Can you work these out from the model? Positions are in its coordinate system, mm. A direction names the side the tool comes from. Give positions to 0.01 mm unless a question says otherwise; leave off trailing zeros. Write each loop counter-clockwise with the first axis right and the second up, starting at its lowest first coordinate (ties: lowest second). Pieces come first, ordered by that corner, then holes.
1. Thinking about a two-plate mould opening in Y: for faces 1 (the cylindrical face through (2.22, 219.61, 609.44)), 2 (the flat face through (-1, 29.618, 320)), 3 (the flat face through (80, 96, 320)), 4 (the flat face through (-1, 274.618, 609)), which applies, pulls with the +Y half, pulls with the -Y half, needs draft (parallel to the pull), parting line crosses it, or undercut?
2. Suppose I cut it at B-B (y = 201.5). Please give me the cut outline in (x, z), and give its area (3 significant figures).
3. Suppose I cut it at A-A (x = 22.5). Please give me the cut outline in (y, z).
4. I'm going to push flat-ended pins straight in: pin 1 (6.5 mm diameter, centred on y = 89.62, z = 140, fed in from +X); pin 2 (6 mm diameter, centred on x = -51, z = 248.5, fed in from +Y); pin 3 (6.5 mm diameter, centred on y = 119.62, z = 410, fed in from -X); pin 4 (12.5 mm diameter, centred on x = 0, y = 229.62, fed in from -Z). Where does each tip first touch, or does it pass through?
5. Suppose I cut it at C-C (z = 178). Please give me the cut outline in (x, y).
6. If I drill on probe 1 along Y at (x, z) = (74, 410); probe 2 along Z at (x, y) = (40, 145.5); probe 3 along Y at (x, z) = (55, 342.5), over which ranges is the centre line in solid material (lowest first)?
7. On a 3-axis mill with a long thin cutter (end or side, diameter ignored), from which of +Z, -Z, +X, -X, +Y, -Y can I reach the whole of each face in a straight line? I mean faces 5 (the flat face through (-1, 213, 570)), 6 (the flat face through (-1, 154, 650)). Say none if no direction works.
```python
from build123d import *

# Parameters (mm, degrees)
SKETCH1_W                    = 160
SKETCH1_H                    = 120
BOSS_EXTRUDE3_DEPTH          = 570
SKETCH4_W                    = 160
SKETCH4_H                    = 245
BOSS_EXTRUDE4_DEPTH          = 80
F_20_5_20_5_DIAMETER_HOLE1_D = 20.5
M8X1_0_TAPPED_HOLE2_D        = 7
M8X1_0_TAPPED_HOLE2_DEPTH    = 20
M8X1_0_TAPPED_HOLE2_TIP      = 2.103012167
M8X1_0_TAPPED_HOLE3_D        = 7
M8X1_0_TAPPED_HOLE3_DEPTH    = 20
M8X1_0_TAPPED_HOLE3_TIP      = 2.103012167
M8X1_0_TAPPED_HOLE1_D        = 7
M8X1_0_TAPPED_HOLE1_DEPTH    = 20
M8X1_0_TAPPED_HOLE1_TIP      = 2.103012167
M12_TAPPED_HOLE1_D           = 10.2
M12_TAPPED_HOLE1_DEPTH       = 30
M12_TAPPED_HOLE1_TIP         = 3.064389157


with BuildPart() as part:
    # Sketch1 → Boss-Extrude3 (new body)
    with BuildSketch(Plane.XY):
        with Locations((0, 89.618320611)):
            Rectangle(SKETCH1_W, SKETCH1_H)
    extrude(amount=BOSS_EXTRUDE3_DEPTH)

    # Sketch4 → Boss-Extrude4 (add)
    with BuildSketch(Plane.XY.offset(570)):
        with Locations((0, 152.118320611)):
            Rectangle(SKETCH4_W, SKETCH4_H)
    extrude(amount=BOSS_EXTRUDE4_DEPTH)

    # Ø20.5 (20.5) Diameter Hole1 (through all)
    with Locations(Plane.XY.offset(650)):
        with Locations((0, 229.618320611)):
            Hole(F_20_5_20_5_DIAMETER_HOLE1_D / 2)

    # M8x1.0 Tapped Hole2
    with Locations(Plane(origin=(0, 149.618320611, 0), x_dir=(1, 0, 0), z_dir=(0, 1, 0))):
        with Locations((-40, -230), (40, -410), (40, -390), (40, -256), (40, -230), (-40, -410), (-40, -390), (-40, -256)):
            Hole(M8X1_0_TAPPED_HOLE2_D / 2, depth=M8X1_0_TAPPED_HOLE2_DEPTH)
            with Locations((0, 0, -(M8X1_0_TAPPED_HOLE2_DEPTH + M8X1_0_TAPPED_HOLE2_TIP / 2))):  # 118° drill point
                Cone(0, M8X1_0_TAPPED_HOLE2_D / 2, M8X1_0_TAPPED_HOLE2_TIP, mode=Mode.SUBTRACT)

    # M8x1.0 Tapped Hole3
    with Locations(Plane(origin=(80, 119.618320611, 140), x_dir=(0, 0, 1), z_dir=(1, 0, 0))):
        with Locations((0, 0), (0, 30), (270, 0), (270, 30)):
            Hole(M8X1_0_TAPPED_HOLE3_D / 2, depth=M8X1_0_TAPPED_HOLE3_DEPTH)
            with Locations((0, 0, -(M8X1_0_TAPPED_HOLE3_DEPTH + M8X1_0_TAPPED_HOLE3_TIP / 2))):  # 118° drill point
                Cone(0, M8X1_0_TAPPED_HOLE3_D / 2, M8X1_0_TAPPED_HOLE3_TIP, mode=Mode.SUBTRACT)

    # M8x1.0 Tapped Hole1
    with Locations(Plane.ZY.offset(80)):
        with Locations((410, 119.618320611), (140, 89.618320611), (410, 89.618320611), (140, 119.618320611)):
            Hole(M8X1_0_TAPPED_HOLE1_D / 2, depth=M8X1_0_TAPPED_HOLE1_DEPTH)
            with Locations((0, 0, -(M8X1_0_TAPPED_HOLE1_DEPTH + M8X1_0_TAPPED_HOLE1_TIP / 2))):  # 118° drill point
                Cone(0, M8X1_0_TAPPED_HOLE1_D / 2, M8X1_0_TAPPED_HOLE1_TIP, mode=Mode.SUBTRACT)

    # M12 Tapped Hole1
    with Locations(Plane(origin=(0, 0, 0), x_dir=(-1, 0, 0), z_dir=(0, 0, -1))):
        with Locations((-50, 119.618320611), (50, 119.618320611), (50, 59.618320611), (-50, 59.618320611)):
            Hole(M12_TAPPED_HOLE1_D / 2, depth=M12_TAPPED_HOLE1_DEPTH)
            with Locations((0, 0, -(M12_TAPPED_HOLE1_DEPTH + M12_TAPPED_HOLE1_TIP / 2))):  # 118° drill point
                Cone(0, M12_TAPPED_HOLE1_D / 2, M12_TAPPED_HOLE1_TIP, mode=Mode.SUBTRACT)


solid = part.part
```
Checks:
1. face 1: undercut
1. face 2: pulls with the -Y half
1. face 3: needs draft
1. face 4: pulls with the +Y half
2. outline: (-80, 570) - (80, 570) - (80, 650) - (-80, 650) - close
2. area: 12,800 mm2
3. outline: (29.62, 0) - (149.62, 0) - (149.62, 570) - (274.62, 570) - (274.62, 650) - (29.62, 650) - close
4. pin 1: stops at x = 59.85
4. pin 2: stops at y = 149.62
4. pin 3: stops at x = -59.85
4. pin 4: passes through
5. outline: (-80, 29.62) - (80, 29.62) - (80, 149.62) - (-80, 149.62) - close
6. probe 1: y = 29.62 to 86.12, 93.12 to 116.12, 123.12 to 149.62
6. probe 2: z = 0 to 226.5, 233.5 to 252.5, 259.5 to 386.5, 393.5 to 406.5, 413.5 to 650
6. probe 3: y = 29.62 to 149.62
7. face 5: -Z, +X, -X, +Y
7. face 6: +Z, +X, -X, +Y, -Y
